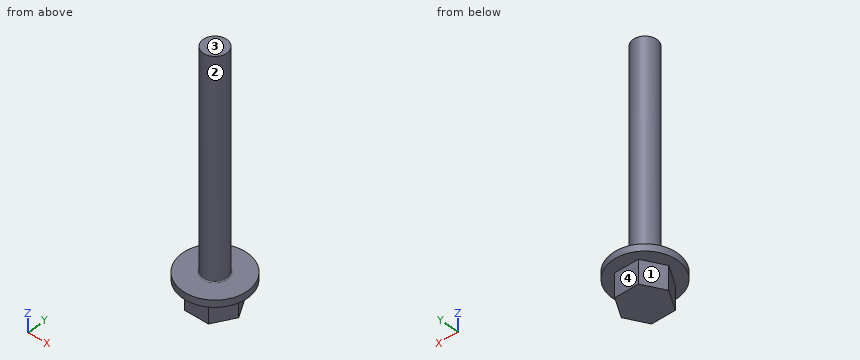
from build123d import *

# Parameters (mm, degrees)
BOSS_EXTRUDE1_DEPTH = 2.794
SKETCH2_R           = 3.81
BOSS_EXTRUDE2_DEPTH = 0.8128
SKETCH3_R           = 1.3843
BOSS_EXTRUDE3_DEPTH = 25.4
FILLET1_R           = 0.1016


with BuildPart() as part:
    # Sketch1 → Boss-Extrude1 (new body)
    with BuildSketch(Plane.XY):
        Polygon((2.756963005, 0), (1.378481503, 2.3876), (-1.378481503, 2.3876), (-2.756963005, 0), (-1.378481503, -2.3876), (1.378481503, -2.3876), align=None)
    extrude(amount=BOSS_EXTRUDE1_DEPTH)

    # Sketch2 → Boss-Extrude2 (add)
    with BuildSketch(Plane.XY.offset(2.794)):
        Circle(SKETCH2_R)
    extrude(amount=BOSS_EXTRUDE2_DEPTH)

    # Sketch3 → Boss-Extrude3 (add)
    with BuildSketch(Plane.XY.offset(3.6068)):
        Circle(SKETCH3_R)
    extrude(amount=BOSS_EXTRUDE3_DEPTH)

    # Fillet1
    fillet1_edges = [part.edges().sort_by_distance(p)[0] for p in [
        (-1.3843, 0, 3.6068),
    ]]
    fillet(fillet1_edges, radius=FILLET1_R)


solid = part.part
Could you check a few things on this model? Use its own coordinates, in mm. Face numbers are marked on the shaded views. A direction names the side the tool comes from. Coordinates: 2 decimals unless noted, no trailing zeros. Loops run counter-clockwise (first coordinate to the right, second up) from the corner with the lowest first, then second, coordinate; pieces in that order, holes last.
1. Imagine slicing it at A-A (x = 0). Please give me the cut outline in (y, z), and give its area (3 significant figures).
2. Imagine slicing it at B-B (z = 12.75). Please give me the cut outline in (x, y), and give its area (3 significant figures).
3. Imagine slicing it at D-D (x = 2). Please give me the cut outline in (y, z), and give its area (3 significant figures).
4. Imagine slicing it at C-C (y = 3.5). Please give me the cut outline in (x, z).
5. For the marked faces 1, 2, 3 and 4, which set-ups out of +Z, -Z, +X, -X, +Y, -Y let a thin tool reach every point of the face, with its end or its side?
6. I need wall thicknesses on L1, parallel to Z at x = 2.25, y = -0.5; L2, parallel to Z at x = -2.75, y = 1; L3, parallel to X at y = -0.25, z = 1.75. Which ranges of each line are inside material? Lowest first, please.
7. For P1, Ø3, axis at x = 2, y = 2.5, coming from the +Z side; P2, Ø2, axis at y = -1, z = 23.5, coming from the +X side; P3, Ø0.8, axis at x = 0.5, z = 1.5, coming from the -Y side; P4, Ø2, axis at y = -3, z = 16, coming from the -X side, each with a flat end and sliding along its axis, tell me the tip position at first contact or that it passes through.
Computed values:
1. outline: (-3.81, 2.79) - (-2.39, 2.79) - (-2.39, 0) - (2.39, 0) - (2.39, 2.79) - (3.81, 2.79) - (3.81, 3.61) - (1.49, 3.61) arc R0.1 cw to (1.38, 3.71) - (1.38, 29.01) - (-1.38, 29.01) - (-1.38, 3.71) arc R0.1 cw to (-1.49, 3.61) - (-3.81, 3.61) - close
1. area: 89.9 mm2
2. outline: circle Ø2.77 at (0, 0)
2. area: 6.02 mm2
3. outline: (-3.24, 2.79) - (-1.31, 2.79) - (-1.31, 0) - (1.31, 0) - (1.31, 2.79) - (3.24, 2.79) - (3.24, 3.61) - (-3.24, 3.61) - close
3. area: 12.6 mm2
4. outline: (-1.51, 2.79) - (1.51, 2.79) - (1.51, 3.61) - (-1.51, 3.61) - close
5. face 1: -Z, -X, +Y
5. face 2: +Z
5. face 3: +Z, +X, -X, +Y, -Y
5. face 4: -Z, +X, -X, +Y
6. L1: z = 0 to 3.61
6. L2: z = 2.79 to 3.61
6. L3: x = -2.61 to 2.61
7. P1: stops at z = 3.61
7. P2: stops at x = 1.38
7. P3: stops at y = -2.39
7. P4: passes through
